```python
from build123d import *

# Parameters (mm, degrees)
BOSS_EXTRUDE1_DEPTH      = 2.5
BOSS_EXTRUDE1_DEPTH_BACK = 2.5
SKETCH1_W                = 54
SKETCH1_H                = 10
SKETCH1_R                = 2.5


with BuildPart() as part:
    # Sketch1 → Boss-Extrude1 (new, two sides: drawn at the far end of the back side and taken through both)
    with BuildSketch(Plane(origin=(0, 0, 0), x_dir=(1, 0, 0), z_dir=(0, 1, 0)).offset(-BOSS_EXTRUDE1_DEPTH_BACK)):
        Rectangle(SKETCH1_W, SKETCH1_H)
        with Locations(Location((-19.5, 0, 0), (0, 0, 270))):
            Circle(SKETCH1_R, mode=Mode.SUBTRACT)
        with Locations(Location((19.5, 0, 0), (0, 0, 270))):
            Circle(SKETCH1_R, mode=Mode.SUBTRACT)
    extrude(amount=BOSS_EXTRUDE1_DEPTH + BOSS_EXTRUDE1_DEPTH_BACK)


solid = part.part
```
For this review, take the finished solid that the model builds, in its own axes (mm). Coordinates: 2 decimals unless noted, no trailing zeros. Write each loop counter-clockwise with the first axis right and the second up, starting at its lowest first coordinate (ties: lowest second). Pieces come first, ordered by that corner, then holes. Notation, with made-up numbers: (-33, -12) - (23, -12) arc R26 ccw to (23, 8) - close; hole circle Ø6 at (57.5, 72). An arc over 180 degrees is marked (long way). Put each result on its own line as item: value.
1. Add section A-A, the plane x = 19.5. Give the boundary of the cut face in (y, z).
Values found:
outline: (-2.5, -5) - (2.5, -5) - (2.5, -2.5) - (-2.5, -2.5) - close; (-2.5, 2.5) - (2.5, 2.5) - (2.5, 5) - (-2.5, 5) - close
2. Mouldability with a two-part tool opening along Z and no side actions: class faces 1 (the flat face through (0, 0, 5)), 2 (the flat face through (0, 2.5, 0)), 3 (the cylindrical face through (22, 0, 0)) as released by +Z, released by -Z, zero draft, split by the parting line, or undercut.
Values found:
face 1: released by +Z
face 2: zero draft
face 3: undercut
3. Add section C-C, the plane z = 0. Give the boundary of the cut face in (x, y).
Values found:
outline: (-27, -2.5) - (-22, -2.5) - (-22, 2.5) - (-27, 2.5) - close; (-17, -2.5) - (17, -2.5) - (17, 2.5) - (-17, 2.5) - close; (22, -2.5) - (27, -2.5) - (27, 2.5) - (22, 2.5) - close
4. Add section B-B, the plane y = 0.4. Give the boundary of the cut face in (x, z), then the cut area to 3 significant figures.
Values found:
outline: (-27, -5) - (27, -5) - (27, 5) - (-27, 5) - close; hole circle Ø5 at (-19.5, 0); hole circle Ø5 at (19.5, 0)
area: 501 mm²
5. Wall thickness on probe 1 along X at (y, z) = (1.1, 0); probe 2 along X at (y, z) = (-1.5, 1.75); probe 3 along Z at (x, y) = (-20, 1.95): over which ranges is each line inside the solid? List them lowest first.
Values found:
probe 1: -27 to -22, -17 to 17, 22 to 27
probe 2: -27 to -21.29, -17.71 to 17.71, 21.29 to 27
probe 3: -5 to -2.45, 2.45 to 5
